Geometry: final body of the model. Coordinates: model frame, mm. A direction names the side the tool comes from. Give positions to 0.01 mm unless a question says otherwise; leave off trailing zeros. Order: outer loops, then holes, each group sorted by start corner. A loop starts at its lowest first (then second) coordinate and runs counter-clockwise, first axis right, second up. Notation, with made-up numbers: (-30, 35.5) -> (6, 35.5) arc R20 cw to (6, 41.5) -> close; hole circle Ø10 at (1, 83). An arc over 180 degrees is marked (long way). Answer in a Markdown table with one row per item. Add a question column.
Q1. Cut plane D-D on z = -3. Return the cut outline in (x, y), and give its area (3 significant figures).
Q2. Cut plane A-A on x = -4.5. Return the cut outline in (y, z), and give its area (3 significant figures).
Q3. Cut plane C-C on y = 1.2. Return the cut outline in (x, z), and give its area (3 significant figures).
Q4. Cut plane B-B on y = 3.4. Return the cut outline in (x, z), and give its area (3 significant figures).
Q5. Line query: line 1 along Z through (x, y) = (0, 1.95); line 2 along X through (y, z) = (1.9, 4.5); line 3 along Z through (x, y) = (-3.75, 0.5). Output: solid intervals per line, ascending. Write a range as from..to.
Q6. Contact query for flat-ended pins moving along their axis: P1, Ø0.8, axis at x = -1, y = 0.5, coming from the +Z side; P2, Ø1.5, axis at y = 1.5, z = -5, coming from the -X side; P3, Ø1.5, axis at y = 3.5, z = -7.5, coming from the -X side. Output: stop coordinate, or through.
Q7. Pull-direction query (X, two-part tool) for faces 1 (the face through (0, 3.5, -6.6)), 2 (the face through (5.4, 3.5, 0)), 3 (the face through (0.6, 3.5, -6)); classes: +X half, -X half, draft (parallel to the pull), parting line (faces both ways), or undercut.
Q8. Set-up query: faces 4 (the face through (-5.4, 3.5, 0)), 5 (the face through (2, 1, 0)), 6 (the face through (5.7, 1.5, 6.1)). Return all of +Z, -Z, +X, -X, +Y, -Y with unobstructed straight access to the full face (end or side cutting, diameter ignored); none if empty.
Autodesk Inventor part; units mm, degrees
ref_plane "YZ Plane" through (0, 0, 0) normal (1, 0, 0) x (0, 1, 0)
ref_plane "XZ Plane" through (0, 0, 0) normal (0, 1, 0) x (-1, 0, 0)
ref_plane "XY Plane" through (0, 0, 0) normal (0, 0, 1) x (1, 0, 0)
sketch "Sketch1" plane through (0, 0, 0) normal (0, 1, 0) x (-1, 0, 0)
  circle A0 centre (0, 0) radius 10
  dimension "d0" = 20
extrude "Extrusion1" add sketch "Sketch1" along normal blind 3
sketch "Sketch2" plane through (0, 3, 0) normal (0, 1, 0) x (1, 0, 0)
  line L0 (-7, -1) -> (-5, -1)
  line L1 (-5, -1) -> (-5, 1)
  line L2 (-5, 1) -> (-7, 1)
  line L3 (-7, 1) -> (-7, -1)
  point P0 (0, 0)
  dimension "d3" = 2
  dimension "d4" = 2
  dimension "d5" = 5
  dimension "d6" = 1
extrude "Extrusion2" add sketch "Sketch2" along normal blind 1
pattern_circular "Circular Pattern2" count 4 over 360 about axis through (0, 0, 0) along (0, 1, 0) of "Extrusion2"
chamfer "Chamfer3" distance 0.9 angle 45 16 edges at (-6, 4, 1) (-5, 4, 0) (-6, 4, -1) (-7, 4, 0) (0, 4, -5) (-1, 4, -6) (0, 4, -7) (1, 4, -6) (6, 4, -1) (7, 4, 0) (5, 4, 0) (6, 4, 1) (1, 4, 6) (-1, 4, 6) (0, 4, 5) (0, 4, 7)
sketch "Sketch3" plane through (0, 3, 0) normal (0, 1, 0) x (1, 0, 0)
  circle A0 centre (-4.5, -4.5) radius 2
  point P0 (0, 0)
  dimension "d24" = 4
  dimension "d25" = 4.5
  dimension "d26" = 4.5
extrude "Extrusion3" cut sketch "Sketch3" against normal through all
pattern_circular "Circular Pattern3" count 4 over 360 about axis through (0, 0, 0) along (0, 1, 0) of "Extrusion3"
sketch "Sketch5" plane through (0, 0, 0) normal (0, -1, 0) x (1, 0, 0)
  line L0 (-2, -2) -> (2, -2)
  line L1 (2, -2) -> (2, 2)
  line L2 (2, 2) -> (-2, 2)
  line L3 (-2, 2) -> (-2, -2)
  point P0 (0, 0)
  dimension "d39" = 4
  dimension "d40" = 4
  dimension "d41" = 2
  dimension "d42" = 2
extrude "Extrusion5" cut sketch "Sketch5" against normal blind 1.5
sketch "Sketch6" plane through (0, 3, 0) normal (0, 1, 0) x (1, 0, 0)
  circle A0 centre (0, 0) radius 1.05
  dimension "d45" = 2.1
extrude "Extrusion6" cut sketch "Sketch6" against normal through all
chamfer "Chamfer4" distance 1 angle 45 1 edges at (-1.05, 3, 0)
properties part number "dent"
Completed:
| question | item | result |
|---|---|---|
| 1 | outline | (-9.54, 0) -> (-5.82, 0) -> (-5.82, 3) -> (-9.54, 3) -> close; (-3.18, 0) -> (3.18, 0) -> (3.18, 3) -> (-3.18, 3) -> close; (5.82, 0) -> (9.54, 0) -> (9.54, 3) -> (5.82, 3) -> close |
| 1 | area | 41.4 mm² |
| 2 | outline | (0, -8.93) -> (3, -8.93) -> (3, -6.5) -> (0, -6.5) -> close; (0, -2.5) -> (3, -2.5) -> (3, 2.5) -> (0, 2.5) -> close; (0, 6.5) -> (3, 6.5) -> (3, 8.93) -> (0, 8.93) -> close |
| 2 | area | 29.6 mm² |
| 3 | outline | circle Ø20 at (0, 0); hole circle Ø4 at (-4.5, -4.5); hole circle Ø4 at (-4.5, 4.5); hole (-2, -2) -> (2, -2) -> (2, 2) -> (-2, 2) -> close; hole circle Ø4 at (4.5, -4.5); hole circle Ø4 at (4.5, 4.5) |
| 3 | area | 248 mm² |
| 4 | outline | (-6.7, -0.7) -> (-5.3, -0.7) -> (-5.3, 0.7) -> (-6.7, 0.7) -> close; (-0.7, -6.7) -> (0.7, -6.7) -> (0.7, -5.3) -> (-0.7, -5.3) -> close; (-0.7, 5.3) -> (0.7, 5.3) -> (0.7, 6.7) -> (-0.7, 6.7) -> close; (5.3, -0.7) -> (6.7, -0.7) -> (6.7, 0.7) -> (5.3, 0.7) -> close |
| 4 | area | 7.84 mm² |
| 5 | line 1 | z = -10..-1.05, 1.05..10 |
| 5 | line 2 | x = -8.93..-6.5, -2.5..2.5, 6.5..8.93 |
| 5 | line 3 | z = -9.27..-6.35, -2.65..2.65, 6.35..9.27 |
| 6 | P1 | stops at z = 9.98 |
| 6 | P2 | stops at x = -9.05 |
| 6 | P3 | stops at x = -7.2 |
| 7 | face 1 | draft |
| 7 | face 2 | undercut |
| 7 | face 3 | +X half |
| 8 | face 4 | +Z, -Z, +Y |
| 8 | face 5 | -Y |
| 8 | face 6 | +Y, -Y |
